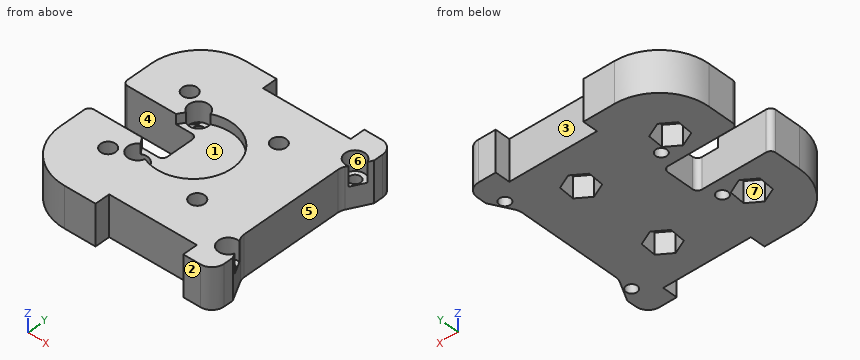
```python
from build123d import *

# Parameters (mm, degrees)
SKETCH_1_W                = 80
SKETCH_1_H                = 80
EXTRUDE_1_DEPTH           = 16.5
FILLET_1_R                = 20
FILLET_2_R                = 5
SKETCH_2_W                = 30
SKETCH_2_H                = 15
CUT_EXTRUDE_1_DEPTH       = 72.127592652
FILLET_3_R                = 2
SKETCH_3_W                = 35.5
SKETCH_3_H                = 6
CUT_EXTRUDE_2_DEPTH       = 72.127592652
SKETCH_4_W                = 35.5
SKETCH_4_H                = 6
CUT_EXTRUDE_3_DEPTH       = 72.127592652
SKETCH_5_W                = 5
SKETCH_5_H                = 44
CUT_EXTRUDE_4_DEPTH       = 72.127592652
HOLE_WIZARD_3_D           = 4.5
HOLE_WIZARD_3_CBORE_D     = 8
HOLE_WIZARD_3_CBORE_DEPTH = 4.6
SKETCH_10_R               = 15.8
CUT_EXTRUDE_5_DEPTH       = 4
SKETCH_18_R               = 4
CUT_EXTRUDE_7_DEPTH       = 8
CUT_EXTRUDE_9_DEPTH       = 72.127592652
FILLET_4_R                = 5
SKETCH_11_R               = 3
CUT_EXTRUDE_10_DEPTH      = 72.127592652
CUT_EXTRUDE_11_DEPTH      = 8.5


with BuildPart() as part:
    # 草图1 → 凸台-拉伸1 (new body)
    with BuildSketch(Plane.XY):
        with Locations((3.759980536, -13.590563907)):
            Rectangle(SKETCH_1_W, SKETCH_1_H)
    extrude(amount=EXTRUDE_1_DEPTH)

    # 圆角1
    fillet_1_edges = [part.edges().sort_by_distance(p)[0] for p in [
        (-36.240019464, 26.409436093, 8.25),
        (-36.240019464, -53.590563907, 8.25),
    ]]
    fillet(fillet_1_edges, radius=FILLET_1_R)

    # 圆角2
    fillet_2_edges = [part.edges().sort_by_distance(p)[0] for p in [
        (43.759980536, 26.409436093, 8.25),
        (43.759980536, -53.590563907, 8.25),
    ]]
    fillet(fillet_2_edges, radius=FILLET_2_R)

    # 草图2 → 切除-拉伸1 (cut, through all)
    with BuildSketch(Plane(origin=(0, 0, 0), x_dir=(-1, 0, 0), z_dir=(0, 0, -1))):
        with Locations((21.240019464, -13.590563907)):
            Rectangle(SKETCH_2_W, SKETCH_2_H)
    extrude(amount=-CUT_EXTRUDE_1_DEPTH, mode=Mode.SUBTRACT)

    # 圆角3
    fillet_3_edges = [part.edges().sort_by_distance(p)[0] for p in [
        (-36.240019464, -6.090563907, 8.25),
        (-36.240019464, -21.090563907, 8.25),
        (-6.240019464, -21.090563907, 8.25),
        (-6.240019464, -6.090563907, 8.25),
    ]]
    fillet(fillet_3_edges, radius=FILLET_3_R)

    # 草图3 → 切除-拉伸2 (cut, through all)
    with BuildSketch(Plane.XY.offset(16.5)):
        with Locations((14.009980536, 23.409436093)):
            Rectangle(SKETCH_3_W, SKETCH_3_H)
    extrude(amount=-CUT_EXTRUDE_2_DEPTH, mode=Mode.SUBTRACT)

    # 草图4 → 切除-拉伸3 (cut, through all)
    with BuildSketch(Plane.XY.offset(16.5)):
        with Locations((14.009980536, -50.590563907)):
            Rectangle(SKETCH_4_W, SKETCH_4_H)
    extrude(amount=-CUT_EXTRUDE_3_DEPTH, mode=Mode.SUBTRACT)

    # 草图5 → 切除-拉伸4 (cut, through all)
    with BuildSketch(Plane.XY.offset(16.5)):
        with Locations((41.259980536, -13.590563907)):
            Rectangle(SKETCH_5_W, SKETCH_5_H)
    extrude(amount=-CUT_EXTRUDE_4_DEPTH, mode=Mode.SUBTRACT)

    # 打孔尺寸(%根据)内六角圆柱头螺钉的类型3 (through all)
    with Locations(Plane.XY.offset(16.5)):
        with Locations((-10.990019464, -0.090563907), (-10.990019464, -27.090563907), (39.009980536, 14.409436093), (39.009980536, -41.590563907)):
            CounterBoreHole(HOLE_WIZARD_3_D / 2, HOLE_WIZARD_3_CBORE_D / 2, HOLE_WIZARD_3_CBORE_DEPTH)

    # 草图10 → 切除-拉伸5 (cut)
    with BuildSketch(Plane.XY.offset(16.5)):
        with Locations((-0.740019464, -13.590563907)):
            Circle(SKETCH_10_R)
    extrude(amount=-CUT_EXTRUDE_5_DEPTH, mode=Mode.SUBTRACT)

    # 草图18 → 切除-拉伸7 (cut)
    with BuildSketch(Plane.XY.offset(16.5)):
        with Locations((-10.990019464, -0.090563907)):
            Circle(SKETCH_18_R)
        with Locations((-10.990019464, -27.090563907)):
            Circle(SKETCH_18_R)
        with Locations((39.009980536, -41.590563907)):
            Circle(SKETCH_18_R)
        with Locations((39.009980536, 14.409436093)):
            Circle(SKETCH_18_R)
    extrude(amount=-CUT_EXTRUDE_7_DEPTH, mode=Mode.SUBTRACT)

    # 草图21 → 切除-拉伸9 (cut, through all)
    with BuildSketch(Plane.XY.offset(16.5)):
        Polygon((38.759980536, 8.409436093), (43.759980536, 17.640880354), (43.759980536, 8.409436093), align=None)
        Polygon((43.759980536, -35.590563907), (38.759980536, -35.590563907), (43.759980536, -44.822008169), align=None)
    extrude(amount=-CUT_EXTRUDE_9_DEPTH, mode=Mode.SUBTRACT)

    # 圆角4
    fillet_4_edges = [part.edges().sort_by_distance(p)[0] for p in [
        (38.759980536, -35.590563907, 8.25),
        (38.759980536, 8.409436093, 8.25),
    ]]
    fillet(fillet_4_edges, radius=FILLET_4_R)

    # 草图11 → 切除-拉伸10 (cut, through all)
    with BuildSketch(Plane.XY.offset(16.5)):
        with Locations((-18.771242384, 4.440659013)):
            Circle(SKETCH_11_R)
        with Locations((17.291203456, 4.440659013)):
            Circle(SKETCH_11_R)
        with Locations((17.291203456, -31.621786828)):
            Circle(SKETCH_11_R)
        with Locations((-18.771242384, -31.621786828)):
            Circle(SKETCH_11_R)
    extrude(amount=-CUT_EXTRUDE_10_DEPTH, mode=Mode.SUBTRACT)

    # 草图22 → 切除-拉伸11 (cut)
    with BuildSketch(Plane(origin=(0, 0, 0), x_dir=(-1, 0, 0), z_dir=(0, 0, -1))):
        Polygon((-16.717600761, 10.765555319), (-22.481922986, 8.099861672), (-23.055525681, 1.774965366), (-17.864806152, -1.884237293), (-12.100483927, 0.781456354), (-11.526881231, 7.10635266), align=None)
        Polygon((-11.526881231, -28.956093181), (-16.717600761, -25.296890522), (-22.481922986, -27.962584169), (-23.055525681, -34.287480475), (-17.864806152, -37.946683134), (-12.100483927, -35.280989487), align=None)
        Polygon((24.535564609, 7.10635266), (19.34484508, 10.765555319), (13.580522855, 8.099861672), (13.006920159, 1.774965366), (18.197639689, -1.884237293), (23.961961914, 0.781456354), align=None)
        Polygon((18.197639689, -37.946683134), (23.961961914, -35.280989487), (24.535564609, -28.956093181), (19.34484508, -25.296890522), (13.580522855, -27.962584169), (13.006920159, -34.287480475), align=None)
    extrude(amount=-CUT_EXTRUDE_11_DEPTH, mode=Mode.SUBTRACT)


solid = part.part
```
The model under review builds one solid part; all positions refer to its coordinate system, in mm. Face numbers are marked on the shaded views. A direction names the side the tool comes from. Round coordinates to 2 decimals unless told otherwise and drop trailing zeros. Loops run counter-clockwise (first coordinate to the right, second up) from the corner with the lowest first, then second, coordinate; pieces in that order, holes last. Notation, with made-up numbers: (12.25, 76) -> (37.25, 76) arc R21 ccw to (37.25, 96) -> close; hole circle Ø4 at (-37.75, 41.5). An arc over 180 degrees is marked (long way). Answer as a JSON object with one key per item and string values. Group by question number.
1) For pin 1 Ø1.5 at (y, z) = (-35, 3) entering from +X; pin 2 Ø5 at (x, z) = (1.5, 10.5) entering from -Y; pin 3 Ø1.5 at (y, z) = (-9, 9) entering from +X, all flat-tipped, find the tip position at first contact; note any pin that passes through.
2) Mouldability with a two-part tool opening along Y and no side actions: class the marked faces 1, 2 and 3 as released by +Y, released by -Y, zero draft, split by the parting line, or undercut.
3) We need section B-B on y = -13. Write out the cut boundary in (x, z), then the cut area to 3 significant figures.
4) For the marked faces 4, 5, 6 and 7, list the 3-axis set-ups (+Z, -Z, +X, -X, +Y, -Y) from which the entire face can be reached by the end or side of a thin tool; tool diameter is ignored.
5) We need section A-A on x = -20.5. Write out the cut boundary in (y, z).
6) We need section D-D on x = 8.5. Write out the cut boundary in (y, z).
7) For line 1 (Y direction, x = -16, z = 1.25) (3 decimals); line 2 (Y direction, x = 13.5, z = 3.75); line 3 (X direction, y = -30, z = 3.75), list the stretches that pass through material, from the lowest coordinate up. Write a range as [from, to].
8) We need section C-C on z = 2. Give the number of separate pieces and of enclosed holes in the cut face, then the cut area to 3 significant figures.
Result set:
{
 "1": {"pin 1": "x = 38.97", "pin 2": "y = -47.59", "pin 3": "x = 38.76"},
 "2": {"face 1": "undercut", "face 2": "released by -Y", "face 3": "released by +Y"},
 "3": {"outline": "(-6.24, 0) -> (38.76, 0) -> (38.76, 16.5) -> (15.05, 16.5) -> (15.05, 12.5) -> (-6.24, 12.5) -> close", "area": "657 mm²"},
 "4": {"face 4": "+Z, -Z, -X", "face 5": "+Z, -Z, +X", "face 6": "+Z", "face 7": "-Z"},
 "5": {"outline": "(-53.13, 0) -> (-36.88, 0) -> (-36.88, 8.5) -> (-34.07, 8.5) -> (-34.07, 16.5) -> (-53.13, 16.5) -> close; (-29.17, 8.5) -> (-26.11, 8.5) -> (-26.11, 0) -> (-21.09, 0) -> (-21.09, 16.5) -> (-29.17, 16.5) -> close; (-6.09, 0) -> (-0.82, 0) -> (-0.82, 8.5) -> (1.99, 8.5) -> (1.99, 16.5) -> (-6.09, 16.5) -> close; (6.89, 8.5) -> (9.95, 8.5) -> (9.95, 0) -> (25.95, 0) -> (25.95, 16.5) -> (6.89, 16.5) -> close"},
 "6": {"outline": "(-47.59, 0) -> (20.41, 0) -> (20.41, 16.5) -> (-0.77, 16.5) -> (-0.77, 12.5) -> (-26.41, 12.5) -> (-26.41, 16.5) -> (-47.59, 16.5) -> close"},
 "7": {"line 1": "[-53.591, -36.397], [-26.844, -21.091], [-6.091, -0.335], [9.219, 26.409]", "line 2": "[-47.59, -35.93], [-27.57, 0.13], [8.5, 20.41]", "line 3": "[-36.24, -24.44], [-13.4, 11.62], [22.67, 38.76]"},
 "8": {"separate pieces": "1", "enclosed holes": "8", "area": "4,590 mm²"}
}
